```python
from build123d import *

# Parameters (mm, degrees)
F1_DEPTH = 55
F2_W     = 4
F2_H     = 5
F3_DEPTH = 58


with BuildPart() as f1:
    # F0 (on Top) → F1 (new body)
    with BuildSketch(Plane.XY):
        Polygon((-50, 4), (-58, -4), (58, -4), (50, 4), align=None)
    extrude(amount=F1_DEPTH)

    # F2 (on Right) → F3 (cut, symmetric)
    with BuildSketch(Plane.YZ):
        with Locations((2, 7.5)):
            Rectangle(F2_W, F2_H)
    extrude(amount=F3_DEPTH, both=True, mode=Mode.SUBTRACT)


solid = f1.part
```
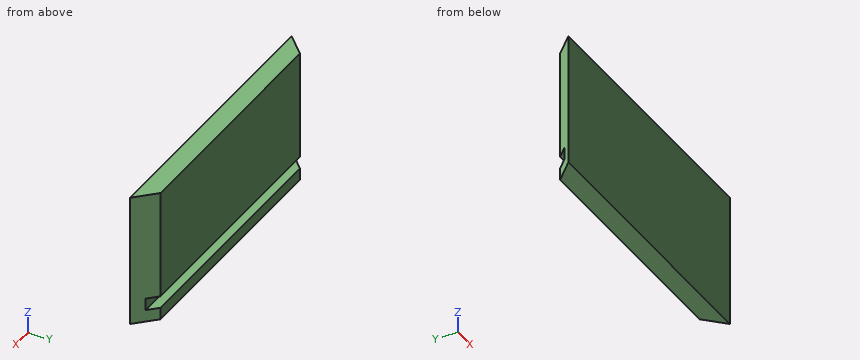
Geometry check sheet. Reference: the model listing, model coordinates, mm. Give positions to 0.01 mm unless a question says otherwise; leave off trailing zeros. Write each loop counter-clockwise with the first axis right and the second up, starting at its lowest first coordinate (ties: lowest second). Pieces come first, ordered by that corner, then holes.
1) Gauge pin test, flat ends, axial feed: pin 1 (4 mm diameter, centred on y = 2.5, z = 29.5, fed in from -X); pin 2 (2 mm diameter, centred on y = -0.5, z = 7.5, fed in from -X); pin 3 (1 mm diameter, centred on y = 0, z = 29, fed in from +X). Record the tip position at first contact, or that the pin passes through.
2) Material ranges on L1, parallel to Z at x = -14.5, y = 0.75; L2, parallel to X at y = 0, z = 52.5; L3, parallel to Y at x = -17, z = 7.5, recorded low to high.
3) Section check A-A, the plane y = 1.75. Record the boundary of the cut face in (x, z).
4) Section check B-B, the plane x = -8. Record the boundary of the cut face in (y, z).
5) Section check D-D, the plane z = 38. Record the boundary of the cut face in (x, y).
6) Section check C-C, the plane z = 8. Record the boundary of the cut face in (x, y).
Computed:
1. pin 1: stops at x = -53.5
1. pin 2: stops at x = -55.5
1. pin 3: stops at x = 54.5
2. L1: z = 0 to 5, 10 to 55
2. L2: x = -54 to 54
2. L3: y = -4 to 0
3. outline: (-52.25, 0) - (52.25, 0) - (52.25, 5) - (-52.25, 5) - close; (-52.25, 10) - (52.25, 10) - (52.25, 55) - (-52.25, 55) - close
4. outline: (-4, 0) - (4, 0) - (4, 5) - (0, 5) - (0, 10) - (4, 10) - (4, 55) - (-4, 55) - close
5. outline: (-58, -4) - (58, -4) - (50, 4) - (-50, 4) - close
6. outline: (-58, -4) - (58, -4) - (54, 0) - (-54, 0) - close
